Part model, mm, in its own coordinate system. Face numbers are marked on the shaded views. Coordinates: 2 decimals unless noted, no trailing zeros. Write each loop counter-clockwise with the first axis right and the second up, starting at its lowest first coordinate (ties: lowest second). Pieces come first, ordered by that corner, then holes. Notation, with made-up numbers: (68.5, 16) - (107.5, 16) arc R16 ccw to (107.5, 29) - close; hole circle Ø3 at (-30, 47.5). An arc over 180 degrees is marked (long way). Write each question's results on one line, items separated by ' | '.
from build123d import *

# Parameters (mm, degrees)
SKETCH_1_R      = 1.35
EXTRUDE_1_DEPTH = 2.3
CHAMFER_1_SIZE  = 0.1


with BuildPart() as part:
    # Эскиз1 → Бобышка-Вытянуть1 (new body)
    with BuildSketch(Plane(origin=(0, 0, 0), x_dir=(1, 0, 0), z_dir=(0, 1, 0))):
        Polygon((3, 0), (1.5, 2.598076211), (-1.5, 2.598076211), (-3, 0), (-1.5, -2.598076211), (1.5, -2.598076211), align=None)
        Circle(SKETCH_1_R, mode=Mode.SUBTRACT)
    extrude(amount=EXTRUDE_1_DEPTH)

    # Фаска1
    chamfer_1_edges = [part.edges().sort_by_distance(p)[0] for p in [
        (0, 2.3, -2.598076211),
        (-2.25, 2.3, -1.299038106),
        (-2.25, 2.3, 1.299038106),
        (-1.35, 0, 0),
        (-1.35, 2.3, 0),
        (0, 2.3, 2.598076211),
        (2.25, 2.3, 1.299038106),
        (0, 0, 2.598076211),
        (-2.25, 0, 1.299038106),
        (-2.25, 0, -1.299038106),
        (2.25, 2.3, -1.299038106),
        (0, 0, -2.598076211),
        (2.25, 0, -1.299038106),
        (2.25, 0, 1.299038106),
    ]]
    chamfer(chamfer_1_edges, length=CHAMFER_1_SIZE)


solid = part.part
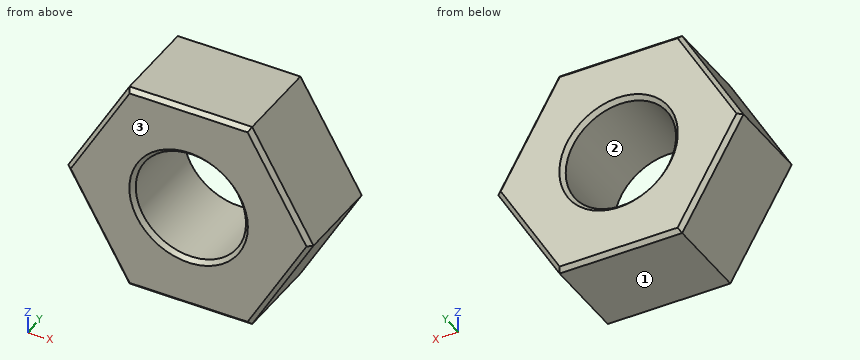
(1) Saw through at A-A on x = 0. Write the cut outline in (y, z), then the cut area to 3 significant figures.
Return value:
outline: (0, -2.5) - (0.1, -2.6) - (2.2, -2.6) - (2.3, -2.5) - (2.3, -1.45) - (2.2, -1.35) - (0.1, -1.35) - (0, -1.45) - close; (0, 1.45) - (0.1, 1.35) - (2.2, 1.35) - (2.3, 1.45) - (2.3, 2.5) - (2.2, 2.6) - (0.1, 2.6) - (0, 2.5) - close | area: 5.70 mm^2
(2) Two-plate mould, pull along Z, no slides. Class the marked faces 1, 2 and 3: released by +Z, released by -Z, zero draft, split by the parting line, or undercut.
Return value:
face 1: released by -Z | face 2: undercut | face 3: zero draft
(3) Saw through at C-C on x = 2.25. Write the cut outline in (y, z).
Return value:
outline: (0, -1.1) - (0.1, -1.3) - (2.2, -1.3) - (2.3, -1.1) - (2.3, 1.1) - (2.2, 1.3) - (0.1, 1.3) - (0, 1.1) - close
(4) Wall check: line 1 (Z direction, x = 0, y = 0.9); line 2 (X direction, y = 0.8, z = 0.05); line 3 (X direction, y = 2.05, z = -2.1). Give the ranges that are in metal, low to high. Write a range as from..to.
Return value:
line 1: z = -2.6..-1.35, 1.35..2.6 | line 2: x = -2.97..-1.35, 1.35..2.97 | line 3: x = -1.79..1.79
(5) Saw through at B-B on y = 2.1. Write the cut outline in (x, z), then the cut area to 3 significant figures.
Return value:
outline: (-3, 0) - (-1.5, -2.6) - (1.5, -2.6) - (3, 0) - (1.5, 2.6) - (-1.5, 2.6) - close; hole circle Ø2.7 at (0, 0) | area: 17.7 mm^2
